For this review, take the finished solid that the model builds, in its own axes (mm). A direction names the side the tool comes from. Round coordinates to 2 decimals unless told otherwise and drop trailing zeros. Order: outer loops, then holes, each group sorted by start corner. A loop starts at its lowest first (then second) coordinate and runs counter-clockwise, first axis right, second up.
```python
from build123d import *

# Parameters (mm, degrees)
SKETCH_W        = 213
SKETCH_H        = 333
PAD_DEPTH       = 12
SKETCH001_R     = 5.2
POCKET_DEPTH    = 5
SKETCH002_R     = 3.2
POCKET001_DEPTH = 7


with BuildPart() as part:
    # Sketch → Pad (new body)
    with BuildSketch(Plane.XY):
        with Locations((106.5, 166.5)):
            Rectangle(SKETCH_W, SKETCH_H)
    extrude(amount=PAD_DEPTH)

    # Sketch001 (on Face6 of Pad) → Pocket (cut)
    with BuildSketch(Plane.XY.offset(12)):
        with Locations((16.5, 264.5)):
            Circle(SKETCH001_R)
        with Locations((16.5, 228.5)):
            Circle(SKETCH001_R)
        with Locations((16.5, 104.5)):
            Circle(SKETCH001_R)
        with Locations((16.5, 68.5)):
            Circle(SKETCH001_R)
        with Locations((196.5, 264.5)):
            Circle(SKETCH001_R)
        with Locations((196.5, 228.5)):
            Circle(SKETCH001_R)
        with Locations((196.5, 104.5)):
            Circle(SKETCH001_R)
        with Locations((196.5, 68.5)):
            Circle(SKETCH001_R)
        with Locations((106.5, 316.5)):
            Circle(SKETCH001_R)
        with Locations((106.5, 16.5)):
            Circle(SKETCH001_R)
    extrude(amount=-POCKET_DEPTH, mode=Mode.SUBTRACT)

    # Sketch002 (on Face23 of Pocket) → Pocket001 (cut)
    with BuildSketch(Plane.XY.offset(7)):
        with Locations((106.5, 316.5)):
            Circle(SKETCH002_R)
        with Locations((16.5, 264.5)):
            Circle(SKETCH002_R)
        with Locations((16.5, 228.5)):
            Circle(SKETCH002_R)
        with Locations((16.5, 104.5)):
            Circle(SKETCH002_R)
        with Locations((16.5, 68.5)):
            Circle(SKETCH002_R)
        with Locations((106.5, 16.5)):
            Circle(SKETCH002_R)
        with Locations((196.5, 68.5)):
            Circle(SKETCH002_R)
        with Locations((196.5, 104.5)):
            Circle(SKETCH002_R)
        with Locations((196.5, 228.5)):
            Circle(SKETCH002_R)
        with Locations((196.5, 264.5)):
            Circle(SKETCH002_R)
    extrude(amount=-POCKET001_DEPTH, mode=Mode.SUBTRACT)


solid = part.part
```
Q1. Take a section at A-A, the plane x = 106.5. State the section outline as (y, z) points, plus the area to 3 significant figures.
Q2. Wall thickness on line 1 (X direction, y = 264.5, z = 8.55); line 2 (Y direction, x = 19, z = 5): over which ranges is each line inside the solid? List them lowest first.
Q3. Take a section at D-D, the plane x = 196.5. Count the separate pieces of the cut face and the enclosed holes in it, plus the area to 3 significant figures.
Q4. Mouldability with a two-part tool opening along Y and no side actions: class faces 1 (the face through (105, 0, 6)), 2 (the face through (13.961, 262.553, 3.549)), 3 (the face through (105, 169, 0)) as +Y half, -Y half, draft (parallel to the pull), parting line (faces both ways), or undercut.
Q5. Tool access review of faces 4 (the face through (191.305, 68.729, 9.535)), 5 (the face through (193.961, 262.553, 3.549)): name each direction out of +Z, -Z, +X, -X, +Y, -Y from which nothing blocks a thin tool from reaching the whole face with its end or side.
Q6. Take a section at B-B, the plane y = 104.5. State the section outline as (x, z) points.
Q7. Clearance check with a flat-ended pin moving along its axis: pin 1 (3 mm diameter, centred on x = 195, y = 229.5, fed in from +Z). State where the tip first meets the part, or that it passes through.
Q8. Take a section at C-C, the plane y = 316.5. State the section outline as (x, z) points.
Working result:
1. outline: (0, 0) - (13.3, 0) - (13.3, 7) - (11.3, 7) - (11.3, 12) - (0, 12) - close; (19.7, 0) - (313.3, 0) - (313.3, 7) - (311.3, 7) - (311.3, 12) - (21.7, 12) - (21.7, 7) - (19.7, 7) - close; (319.7, 0) - (333, 0) - (333, 12) - (321.7, 12) - (321.7, 7) - (319.7, 7) - close
1. area: 3,800 mm2
2. line 1: x = 0 to 11.3, 21.7 to 191.3, 201.7 to 213
2. line 2: y = 0 to 66.5, 70.5 to 102.5, 106.5 to 226.5, 230.5 to 262.5, 266.5 to 333
3. separate pieces: 5
3. enclosed holes: 0
3. area: 3,610 mm2
4. face 1: -Y half
4. face 2: undercut
4. face 3: draft
5. face 4: +Z
5. face 5: +Z, -Z
6. outline: (0, 0) - (13.3, 0) - (13.3, 7) - (11.3, 7) - (11.3, 12) - (0, 12) - close; (19.7, 0) - (193.3, 0) - (193.3, 7) - (191.3, 7) - (191.3, 12) - (21.7, 12) - (21.7, 7) - (19.7, 7) - close; (199.7, 0) - (213, 0) - (213, 12) - (201.7, 12) - (201.7, 7) - (199.7, 7) - close
7. pin 1: stops at z = 7
8. outline: (0, 0) - (103.3, 0) - (103.3, 7) - (101.3, 7) - (101.3, 12) - (0, 12) - close; (109.7, 0) - (213, 0) - (213, 12) - (111.7, 12) - (111.7, 7) - (109.7, 7) - close
